Geometry check sheet. Reference: the model listing, model coordinates, mm. Face numbers are marked on the shaded views. Round coordinates to 2 decimals unless told otherwise and drop trailing zeros. Loops run counter-clockwise (first coordinate to the right, second up) from the corner with the lowest first, then second, coordinate; pieces in that order, holes last. Notation, with made-up numbers: (27.25, -38) - (37.25, -38) arc R36 cw to (37.25, -1) - close; hole circle Ø1 at (-16, 40). An arc over 180 degrees is marked (long way). Answer as CSV lines item,"result". Start each with the question number.
1) Depth check by flat-ended pin: P1, Ø1.3, axis at x = -28.5, z = 38, coming from the -Y side; P2, Ø7.5, axis at x = -2.5, y = -16.5, coming from the +Z side; P3, Ø7.5, axis at y = -13.5, z = -9.5, coming from the -X side. Enter the tip coordinate at first touch or a pass-through.
2) Draft check along X on the marked faces 1, 2, 3 and 4. Enter one of: released by +X, released by -X, zero draft, split by the parting line, or undercut.
3) Cross-section at B-B on x = 7.5. Record the boundary of the cut face in (y, z), and give its area (3 significant figures).
4) Thickness scan on line 1 along Y through (x, z) = (-11.5, 34.5); line 2 along X through (y, z) = (-10.25, -30.5); line 3 along Z through (x, y) = (-9.5, -7.25). Record the ranges inside material, lowest first.
5) Cross-section at A-A on z = 12.5. Record the boundary of the cut face in (x, y).
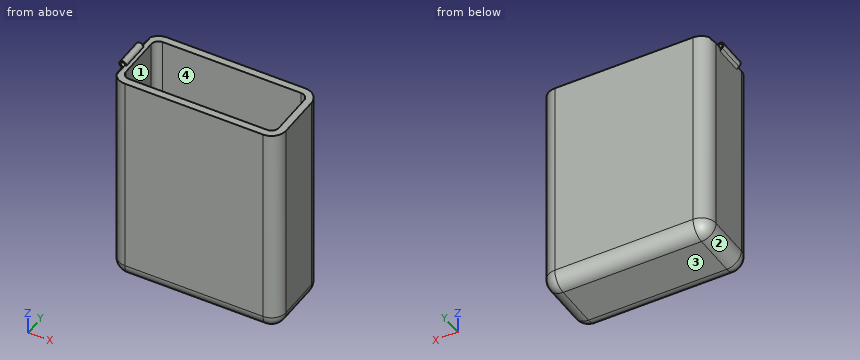
from build123d import *

# Parameters (mm, degrees)
F0_W     = 58.42
F0_H     = 76.2
F1_DEPTH = 25.4
F2_R     = 5.08
F3_T     = -2.54
F5_R     = 1.27
F6_DEPTH = 5.08
F7_R     = 1.27
F8_R     = 0.762
F9_DEPTH = 76.2


with BuildPart() as f1:
    # F0 (on Front) → F1 (new body)
    with BuildSketch(Plane.XZ):
        Rectangle(F0_W, F0_H)
    extrude(amount=F1_DEPTH)

    # F2
    f2_edges = [f1.edges().sort_by_distance(p)[0] for p in [
        (-29.21, -25.4, 0),
        (29.21, -25.4, 0),
        (29.21, 0, 0),
        (-29.21, 0, 0),
        (-29.21, -12.7, -38.1),
        (29.21, -12.7, -38.1),
        (0, 0, -38.1),
        (0, -25.4, -38.1),
    ]]
    fillet(f2_edges, radius=F2_R)

    # F3
    f3_openings = [f1.faces().sort_by_distance(p)[0] for p in [
        (0, -12.7, 38.1),
    ]]
    offset(amount=F3_T, openings=f3_openings)

    # F5 (on offset) → F6 (join, symmetric)
    with BuildSketch(Plane(origin=(0, -12.7, 0), x_dir=(-1, 0, 0), z_dir=(0, 1, 0))):
        with Locations((29.21, 38.1)):
            Circle(F5_R)
    extrude(amount=F6_DEPTH, both=True)

    # F7
    f7_edges = [f1.edges().sort_by_distance(p)[0] for p in [
        (-29.21, -12.7, 36.83),
    ]]
    fillet(f7_edges, radius=F7_R)

    # F8 (on face) → F9 (cut, symmetric)
    with BuildSketch(Plane(origin=(0, -7.62, 0), x_dir=(-1, 0, 0), z_dir=(0, 1, 0))):
        with Locations((29.21, 38.1)):
            Circle(F8_R)
    extrude(amount=F9_DEPTH, both=True, mode=Mode.SUBTRACT)


solid = f1.part
Answer block:
1,P1,"stops at y = -23.78"
1,P2,"stops at z = -35.56"
1,P3,"stops at x = -29.21"
2,face 1,"undercut"
2,face 2,"released by -X"
2,face 3,"zero draft"
2,face 4,"undercut"
3,outline,"(-25.4, -33.02) arc R5.08 ccw to (-20.32, -38.1) - (-5.08, -38.1) arc R5.08 ccw to (0, -33.02) - (0, 38.1) - (-2.54, 38.1) - (-2.54, -33.02) arc R2.54 cw to (-5.08, -35.56) - (-20.32, -35.56) arc R2.54 cw to (-22.86, -33.02) - (-22.86, 38.1) - (-25.4, 38.1) - close"
3,area,"430 mm^2"
4,line 1,"y = -25.4 to -22.86, -2.54 to 0"
4,line 2,"x = -29.21 to -26.67, 26.67 to 29.21"
4,line 3,"z = -38.1 to -35.56"
5,outline,"(-29.21, -20.32) arc R5.08 ccw to (-24.13, -25.4) - (24.13, -25.4) arc R5.08 ccw to (29.21, -20.32) - (29.21, -5.08) arc R5.08 ccw to (24.13, 0) - (-24.13, 0) arc R5.08 ccw to (-29.21, -5.08) - close; hole (-26.67, -20.32) arc R2.54 ccw to (-24.13, -22.86) - (24.13, -22.86) arc R2.54 ccw to (26.67, -20.32) - (26.67, -5.08) arc R2.54 ccw to (24.13, -2.54) - (-24.13, -2.54) arc R2.54 ccw to (-26.67, -5.08) - close"
